Here's how the part is built. I have some questions about the finished solid (model axes, mm). Face numbers are marked on the shaded views. Round coordinates to 2 decimals unless told otherwise and drop trailing zeros. Order: outer loops, then holes, each group sorted by start corner. A loop starts at its lowest first (then second) coordinate and runs counter-clockwise, first axis right, second up. Notation, with made-up numbers: (-27, -25) - (-16, -25) arc R29 cw to (-16, 14) - close; hole circle Ø10 at (61, 23). An arc over 180 degrees is marked (long way). One line per item, written item: value.
from build123d import *

# Parameters (mm, degrees)
SKETCH3_R                 = 6.7437
BASE_FLANGE1_DEPTH        = 3.4163
EDGE_FLANGE1_DEPTH        = 120.765617952
EDGE_FLANGE1_BEND_DEPTH   = 120.765617952
EDGE_FLANGE1_BEND_2_DEPTH = 120.765617952
EDGE_FLANGE1_BEND_3_DEPTH = 120.765617952


# Sheet-metal steps are written as plain solids
with BuildPart() as part:
    # Sketch3 → Base-Flange1 (new body)
    with BuildSketch(Plane(origin=(0, 0, 0), x_dir=(1, 0, 0), z_dir=(0, 1, 0))):
        with BuildLine():
            Line((-60.382808976, 81.5594), (60.382808976, 81.5594))
            ThreePointArc((60.382808976, 81.5594), (64.390963201, 64.390963201), (81.5594, 60.382808976))
            Line((81.5594, 60.382808976), (81.5594, -60.382808976))
            ThreePointArc((81.5594, -60.382808976), (64.390963201, -64.390963201), (60.382808976, -81.5594))
            Line((60.382808976, -81.5594), (-60.382808976, -81.5594))
            ThreePointArc((-60.382808976, -81.5594), (-64.390963201, -64.390963201), (-81.5594, -60.382808976))
            Line((-81.5594, -60.382808976), (-81.5594, 60.382808976))
            ThreePointArc((-81.5594, 60.382808976), (-64.390963201, 64.390963201), (-60.382808976, 81.5594))
        make_face()
        with Locations(Location((0, 0, 0), (0, 0, 270))):
            Circle(SKETCH3_R, mode=Mode.SUBTRACT)
    extrude(amount=-BASE_FLANGE1_DEPTH)

    # Edge-Flange1 section (across the edge) → Edge-Flange1 (add)
    with BuildSketch(Plane(origin=(60.382808976, -3.4163, 82.296), x_dir=(0, 0, -1), z_dir=(-1, 0, 0))):
        with BuildLine():
            Line((-3.4163, 0.7366), (-3.4163, 15.6337))
            Line((-3.4163, 15.6337), (0, 15.6337))
            Line((0, 15.6337), (0, 0.7366))
            ThreePointArc((0, 0.7366), (0.215745145, 0.215745145), (0.7366, 0))
            Line((0.7366, 0), (0.7366, -3.4163))
            ThreePointArc((0.7366, -3.4163), (-2.199943752, -2.199943752), (-3.4163, 0.7366))
        make_face()
    extrude(amount=EDGE_FLANGE1_DEPTH)

    # Edge-Flange1 section 2 (across the edge) → Edge-Flange1 bend (add)
    with BuildSketch(Plane(origin=(82.296, -3.4163, -60.382808976), x_dir=(-1, 0, 0), z_dir=(0, 0, 1))):
        with BuildLine():
            Line((-3.4163, 0.7366), (-3.4163, 15.6337))
            Line((-3.4163, 15.6337), (0, 15.6337))
            Line((0, 15.6337), (0, 0.7366))
            ThreePointArc((0, 0.7366), (0.215745145, 0.215745145), (0.7366, 0))
            Line((0.7366, 0), (0.7366, -3.4163))
            ThreePointArc((0.7366, -3.4163), (-2.199943752, -2.199943752), (-3.4163, 0.7366))
        make_face()
    extrude(amount=EDGE_FLANGE1_BEND_DEPTH)

    # Edge-Flange1 section 3 (across the edge) → Edge-Flange1 bend 2 (add)
    with BuildSketch(Plane(origin=(-60.382808976, -3.4163, -82.296), x_dir=(0, 0, 1), z_dir=(1, 0, 0))):
        with BuildLine():
            Line((-3.4163, 0.7366), (-3.4163, 15.6337))
            Line((-3.4163, 15.6337), (0, 15.6337))
            Line((0, 15.6337), (0, 0.7366))
            ThreePointArc((0, 0.7366), (0.215745145, 0.215745145), (0.7366, 0))
            Line((0.7366, 0), (0.7366, -3.4163))
            ThreePointArc((0.7366, -3.4163), (-2.199943752, -2.199943752), (-3.4163, 0.7366))
        make_face()
    extrude(amount=EDGE_FLANGE1_BEND_2_DEPTH)

    # Edge-Flange1 section 4 (across the edge) → Edge-Flange1 bend 3 (add)
    with BuildSketch(Plane(origin=(-82.296, -3.4163, 60.382808976), x_dir=(1, 0, 0), z_dir=(0, 0, -1))):
        with BuildLine():
            Line((-3.4163, 0.7366), (-3.4163, 15.6337))
            Line((-3.4163, 15.6337), (0, 15.6337))
            Line((0, 15.6337), (0, 0.7366))
            ThreePointArc((0, 0.7366), (0.215745145, 0.215745145), (0.7366, 0))
            Line((0.7366, 0), (0.7366, -3.4163))
            ThreePointArc((0.7366, -3.4163), (-2.199943752, -2.199943752), (-3.4163, 0.7366))
        make_face()
    extrude(amount=EDGE_FLANGE1_BEND_3_DEPTH)


solid = part.part
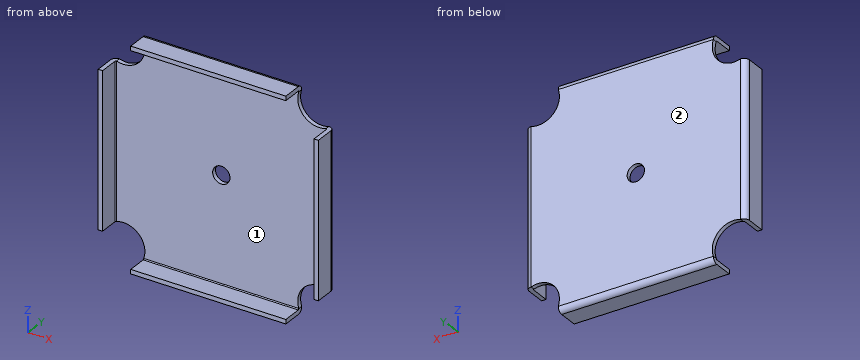
Q1. We'd pull the mould along Z, two halves only. Please class the marked faces 1 and 2: released by +Z, released by -Z, zero draft, split by the parting line, or undercut.
Results list:
face 1: undercut
face 2: zero draft
Q2. If I drill on line 1 along X through (y, z) = (-15, -20); line 2 along Y through (x, z) = (-64, -29), over which ranges is the centre line in solid material (lowest first)?
Results list:
line 1: -85.71 to -82.3, 82.3 to 85.71
line 2: -3.42 to 0
Q3. If we section it at C-C, the plane z = 0: Please give me the cut outline in (x, y).
Results list:
outline: (-85.71, -19.05) - (-82.3, -19.05) - (-82.3, -4.15) arc R0.74 cw to (-81.56, -3.42) - (-6.74, -3.42) - (-6.74, 0) - (-81.56, 0) arc R4.15 ccw to (-85.71, -4.15) - close; (6.74, -3.42) - (81.56, -3.42) arc R0.74 cw to (82.3, -4.15) - (82.3, -19.05) - (85.71, -19.05) - (85.71, -4.15) arc R4.15 ccw to (81.56, 0) - (6.74, 0) - close
Q4. If we section it at B-B, the plane x = 0: Please give me the cut outline in (y, z), then the cut area to 3 significant figures.
Results list:
outline: (-19.05, -85.71) - (-4.15, -85.71) arc R4.15 ccw to (0, -81.56) - (0, -6.74) - (-3.42, -6.74) - (-3.42, -81.56) arc R0.74 cw to (-4.15, -82.3) - (-19.05, -82.3) - close; (-19.05, 82.3) - (-4.15, 82.3) arc R0.74 cw to (-3.42, 81.56) - (-3.42, 6.74) - (0, 6.74) - (0, 81.56) arc R4.15 ccw to (-4.15, 85.71) - (-19.05, 85.71) - close
area: 639 mm²
Q5. Will these pins go through, and if not, where does the flat tip stop? pin 1 (10 mm diameter, centred on x = -17.5, z = -36, fed in from -Y); pin 2 (4.5 mm diameter, centred on x = -84.5, y = -9.5, fed in from -Z); pin 3 (1.2 mm diameter, centred on y = -11, z = -82.5, fed in from -X); pin 4 (12 mm diameter, centred on x = 0, z = 0, fed in from -Y).
Results list:
pin 1: y = -3.42
pin 2: z = -60.38
pin 3: x = -60.38
pin 4: through
Q6. If we section it at D-D, the plane z = 48: Please give me the cut outline in (x, y), then the cut area to 3 significant figures.
Results list:
outline: (-85.71, -19.05) - (-82.3, -19.05) - (-82.3, -4.15) arc R0.74 cw to (-81.56, -3.42) - (81.56, -3.42) arc R0.74 cw to (82.3, -4.15) - (82.3, -19.05) - (85.71, -19.05) - (85.71, -4.15) arc R4.15 ccw to (81.56, 0) - (-81.56, 0) arc R4.15 ccw to (-85.71, -4.15) - close
area: 685 mm²
Q7. If we section it at A-A, the plane y = -6.25: Please give me the cut outline in (x, z).
Results list:
outline: (-85.71, -60.38) - (-82.3, -60.38) - (-82.3, 60.38) - (-85.71, 60.38) - close; (-60.38, -85.71) - (60.38, -85.71) - (60.38, -82.3) - (-60.38, -82.3) - close; (-60.38, 82.3) - (60.38, 82.3) - (60.38, 85.71) - (-60.38, 85.71) - close; (82.3, -60.38) - (85.71, -60.38) - (85.71, 60.38) - (82.3, 60.38) - close
